from build123d import *

# Parameters (mm, degrees)
F2_R    = 5
F3_SIZE = 1


with BuildPart() as f1:
    # F0 (on Front) → F1 (revolve)
    with BuildSketch(Plane.XZ):
        Polygon((2.5, 52), (2.5, 0), (5, 0), (5, 50), (8, 50), (8, 52), align=None)
    revolve(axis=Axis((0, 0, 22.814085), (0, 0, -1)))

    # F2
    f2_edges = [f1.edges().sort_by_distance(p)[0] for p in [
        (-2.5, 0, 52),
    ]]
    fillet(f2_edges, radius=F2_R)

    # F3
    f3_edges = [f1.edges().sort_by_distance(p)[0] for p in [
        (-5, 0, 0),
    ]]
    chamfer(f3_edges, length=F3_SIZE)


solid = f1.part
Geometry check sheet. Reference: the model listing, model coordinates, mm. A direction names the side the tool comes from. Round coordinates to 2 decimals unless told otherwise and drop trailing zeros. Write each loop counter-clockwise with the first axis right and the second up, starting at its lowest first coordinate (ties: lowest second). Pieces come first, ordered by that corner, then holes. Notation, with made-up numbers: (75.5, 40.5) -> (93.5, 40.5) arc R23 ccw to (93.5, 77.5) -> close; hole circle Ø4 at (2.5, 15). An arc over 180 degrees is marked (long way). One line per item, written item: value. Start each with the question number.
(1) Cross-section at C-C, the plane z = 5. Record the cut outline in (x, y).
(2) Go/stop test with flat-tipped pins: pin 1 Ø2 at (x, y) = (-6, 2.5) entering from -Z; pin 2 Ø1 at (x, y) = (3, -5) entering from +Z; pin 3 Ø2 at (x, y) = (1.5, 5) entering from +Z. Record where each tip stops, or that it passes through.
(3) Access from +Z, -Z, +X, -X, +Y, -Y to the whole of each face (thin tool, end or side, straight path). Record for faces 4 (the flat face through (-2, -2, 0)), 5 (the cylindrical face through (-1.08, 4.88, 25.84)).
(4) Cross-section at A-A, the plane y = 0. Record the cut outline in (x, z).
(5) Scan lines: line 1 (X direction, y = 0, z = 26); line 2 (X direction, y = -1.5, z = 15.5). Record each from-to range of solid material in increasing order. Write a range as [from, to].
(6) Draft check along X on faces 1 (the cylindrical face through (-0.54, 2.44, 23.17)), 2 (the cylindrical face through (-1.73, 7.81, 51.01)), 3 (the flat face through (0.1, 5.2, 50)). Enter one of: +X half, -X half, draft (parallel to the pull), parting line (faces both ways), or undercut.
Answer:
1. outline: circle Ø10 at (0, 0); hole circle Ø5 at (0, 0)
2. pin 1: z = 50
2. pin 2: z = 51.86
2. pin 3: z = 51.83
3. face 4: -Z, +X, -X, +Y, -Y
3. face 5: -Z
4. outline: (-8, 50) -> (-5, 50) -> (-5, 1) -> (-4, 0) -> (-2.5, 0) -> (-2.5, 47) arc R5 ccw to (-7.5, 52) -> (-8, 52) -> close; (2.5, 0) -> (4, 0) -> (5, 1) -> (5, 50) -> (8, 50) -> (8, 52) -> (7.5, 52) arc R5 ccw to (2.5, 47) -> close
5. line 1: [-5, -2.5], [2.5, 5]
5. line 2: [-4.77, -2], [2, 4.77]
6. face 1: undercut
6. face 2: parting line
6. face 3: draft
